Geometry check sheet. Reference: the model listing, model coordinates, mm. Face numbers are marked on the shaded views. A direction names the side the tool comes from. Give positions to 0.01 mm unless a question says otherwise; leave off trailing zeros. Loops run counter-clockwise (first coordinate to the right, second up) from the corner with the lowest first, then second, coordinate; pieces in that order, holes last. Notation, with made-up numbers: (28.25, 34) -> (56.25, 34) arc R16 cw to (56.25, 42) -> close; hole circle Ø1 at (-24.75, 22.5). An arc over 180 degrees is marked (long way). One line per item, written item: value. Start each with the question number.
(1) Sectioned sample at D-D, the plane z = 1.65. Record the cut outline in (x, y).
(2) Gauge pin test, flat ends, axial feed: pin 1 Ø4 at (x, y) = (3.5, -2.5) entering from +Z; pin 2 Ø2 at (x, z) = (0, 3.5) entering from +Y; pin 3 Ø5 at (x, y) = (-3.5, -2.5) entering from +Z. Record the tip position at first contact, or that the pin passes through.
(3) Sectioned sample at C-C, the plane z = 4.1. Record the cut outline in (x, y), then the cut area to 3 significant figures.
(4) Sectioned sample at A-A, the plane x = 0. Record the cut outline in (y, z), then the cut area to 3 significant figures.
(5) Scan lines: line 1 along Z through (x, y) = (3, 2.75); line 2 along X through (y, z) = (4, 0.7); line 3 along Y through (x, z) = (-1.75, 1.5). Record each from-to range of solid material in increasing order. Write a range as from..to.
(6) Tool access check on the marked faces 1 and 2. Record the directions out of +Z, -Z, +X, -X, +Y, -Y that give a thin tool (end or side, any length) a straight path to the whole face; none if there is none.
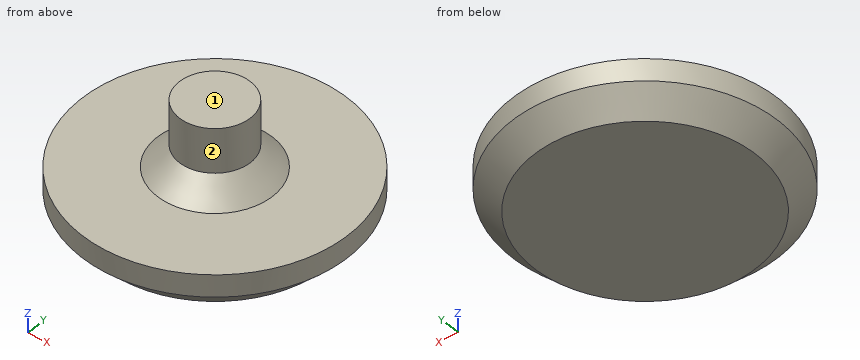
from build123d import *

# Parameters (mm, degrees)
F0_R     = 6
F0_R_2   = 1.6
F1_DEPTH = 2
F2_DEPTH = 5
F3_SIZE  = 1


with BuildPart() as f1:
    # F0 (on Top) → F1 (new body)
    with BuildSketch(Plane.XY):
        Circle(F0_R)
        Circle(F0_R_2, mode=Mode.SUBTRACT)
    extrude(amount=F1_DEPTH)

    # F0 (on Top) → F2 (join)
    with BuildSketch(Plane.XY):
        Circle(F0_R_2)
    extrude(amount=F2_DEPTH)

    # F3
    f3_edges = [f1.edges().sort_by_distance(p)[0] for p in [
        (-6, 0, 0),
        (-1.6, 0, 2),
    ]]
    chamfer(f3_edges, length=F3_SIZE)


solid = f1.part
Calculated:
1. outline: circle Ø12 at (0, 0)
2. pin 1: stops at z = 2.3
2. pin 2: stops at y = 2.1
2. pin 3: stops at z = 2.8
3. outline: circle Ø3.2 at (0, 0)
3. area: 8.04 mm2
4. outline: (-6, 1) -> (-5, 0) -> (5, 0) -> (6, 1) -> (6, 2) -> (2.6, 2) -> (1.6, 3) -> (1.6, 5) -> (-1.6, 5) -> (-1.6, 3) -> (-2.6, 2) -> (-6, 2) -> close
4. area: 33.6 mm2
5. line 1: z = 0..2
5. line 2: x = -4.06..4.06
5. line 3: y = -5.74..5.74
6. face 1: +Z, +X, -X, +Y, -Y
6. face 2: +Z
